Geometry check sheet. Reference: the model listing, model coordinates, mm. A direction names the side the tool comes from. Give positions to 0.01 mm unless a question says otherwise; leave off trailing zeros. Loops run counter-clockwise (first coordinate to the right, second up) from the corner with the lowest first, then second, coordinate; pieces in that order, holes last.
1. Release check for a two-part mould opening along Y. For faces 4 (the cylindrical face through (-43.28, -11.49, 15.55)), 5 (the flat face through (-41, -18, 15)), 6 (the cylindrical face through (-43.306, -11.894, 17.398)), 7 (the flat face through (-42.292, -9, 15)) record: +Y half, -Y half, draft (parallel to the pull), parting line (faces both ways), or undercut.
2. Go/stop test with flat-tipped pins: pin 1 Ø1.2 at (y, z) = (-12, 15) entering from -X; pin 2 Ø3 at (x, y) = (-36.29, -12) entering from -Z; pin 3 Ø1.5 at (y, z) = (-9.5, 14.5) entering from +X; pin 4 Ø1 at (y, z) = (-7.5, 18) entering from -X. Record where each tip stops, or that it passes through.
3. Cross-section at C-C, the plane y = -12. Record the cut outline in (x, z).
4. Cross-section at A-A, the plane z = 18. Record the cut outline in (x, y).
5. Tool access check on faces 1 (the flat face through (-33.292, -12, 12)), 2 (the flat face through (-40.792, -12, 15)), 3 (the flat face through (-42.242, -12, 15)). Record the directions out of +Z, -Z, +X, -X, +Y, -Y that give a thin tool (end or side, any length) a straight path to the whole face; none if there is none.
6. Material ranges on L1, parallel to Y at x = -36.25, z = 11.5; L2, parallel to Z at x = -34, y = -10; L3, parallel to Y at x = -42.95, z = 15, recorded low to high.
7. Cross-section at D-D, the plane z = 15. Record the cut outline in (x, y), plus the area to 3 significant figures.
8. Cross-section at B-B, the plane x = -34.25. Record the cut outline in (y, z), plus the area to 3 significant figures.
from build123d import *

# Parameters (mm, degrees)
SPRING_FRONT_CABLE_CLEVIS_1_SKETCH_W  = 1.5
SPRING_FRONT_CABLE_CLEVIS_1_SKETCH_H  = 12
SPRING_FRONT_CABLE_CLEVIS_1_DEPTH     = 8.1
SPRING_FRONT_CLEVIS_1_LOWER_SKETCH_W  = 7.6
SPRING_FRONT_CLEVIS_1_LOWER_SKETCH_H  = 12
SPRING_FRONT_CLEVIS_1_LOWER_DEPTH     = 1.5
SPRING_FRONT_CLEVIS_1_UPPER_SKETCH_W  = 7.6
SPRING_FRONT_CLEVIS_1_UPPER_SKETCH_H  = 12
SPRING_FRONT_CLEVIS_1_UPPER_DEPTH     = 1.6
FRONT_CLEVIS_SWAGE_HOUSING_1_SKETCH_R = 2.4
FRONT_CLEVIS_SWAGE_HOUSING_1_DEPTH    = 2.1
FRONT_CLEVIS_SWAGE_BORE_1_SKETCH_R    = 0.75
FRONT_CLEVIS_SWAGE_BORE_1_DEPTH       = 2.15
FRONT_CLEVIS_PIN_BORE_1_SKETCH_R      = 1.6
FRONT_CLEVIS_PIN_BORE_1_DEPTH         = 8.3


with BuildPart() as part:
    # Spring Front Cable Clevis 1 sketch → Spring Front Cable Clevis 1 (new body)
    with BuildSketch(Plane.XY.offset(11)):
        with Locations((-41.541651246, -12)):
            Rectangle(SPRING_FRONT_CABLE_CLEVIS_1_SKETCH_W, SPRING_FRONT_CABLE_CLEVIS_1_SKETCH_H)
    extrude(amount=SPRING_FRONT_CABLE_CLEVIS_1_DEPTH)

    # Spring Front Clevis 1 Lower sketch → Spring Front Clevis 1 Lower (add)
    with BuildSketch(Plane.XY.offset(11)):
        with Locations((-37.091651246, -12)):
            Rectangle(SPRING_FRONT_CLEVIS_1_LOWER_SKETCH_W, SPRING_FRONT_CLEVIS_1_LOWER_SKETCH_H)
    extrude(amount=SPRING_FRONT_CLEVIS_1_LOWER_DEPTH)

    # Spring Front Clevis 1 Upper sketch → Spring Front Clevis 1 Upper (add)
    with BuildSketch(Plane.XY.offset(17.5)):
        with Locations((-37.091651246, -12)):
            Rectangle(SPRING_FRONT_CLEVIS_1_UPPER_SKETCH_W, SPRING_FRONT_CLEVIS_1_UPPER_SKETCH_H)
    extrude(amount=SPRING_FRONT_CLEVIS_1_UPPER_DEPTH)

    # Front Clevis Swage Housing 1 sketch → Front Clevis Swage Housing 1 (add)
    with BuildSketch(Plane(origin=(-44.291651246, 0, 0), x_dir=(0, 0, -1), z_dir=(1, 0, 0))):
        with Locations((-15, -12)):
            Circle(FRONT_CLEVIS_SWAGE_HOUSING_1_SKETCH_R)
    extrude(amount=FRONT_CLEVIS_SWAGE_HOUSING_1_DEPTH)

    # Front Clevis Swage Bore 1 sketch → Front Clevis Swage Bore 1 (cut)
    with BuildSketch(Plane(origin=(-44.391651246, 0, 0), x_dir=(0, 0, -1), z_dir=(1, 0, 0))):
        with Locations((-15, -12)):
            Circle(FRONT_CLEVIS_SWAGE_BORE_1_SKETCH_R)
    extrude(amount=FRONT_CLEVIS_SWAGE_BORE_1_DEPTH, mode=Mode.SUBTRACT)

    # Front Clevis Pin Bore 1 sketch → Front Clevis Pin Bore 1 (cut)
    with BuildSketch(Plane.XY.offset(10.9)):
        with Locations((-36.291651246, -12)):
            Circle(FRONT_CLEVIS_PIN_BORE_1_SKETCH_R)
    extrude(amount=FRONT_CLEVIS_PIN_BORE_1_DEPTH, mode=Mode.SUBTRACT)


solid = part.part
Result:
1. face 4: undercut
1. face 5: -Y half
1. face 6: parting line
1. face 7: draft
2. pin 1: stops at x = -42.24
2. pin 2: passes through
2. pin 3: stops at x = -40.79
2. pin 4: stops at x = -42.29
3. outline: (-44.29, 12.6) - (-42.29, 12.6) - (-42.29, 11) - (-37.89, 11) - (-37.89, 12.5) - (-40.79, 12.5) - (-40.79, 17.5) - (-37.89, 17.5) - (-37.89, 19.1) - (-42.29, 19.1) - (-42.29, 17.4) - (-44.29, 17.4) - (-44.29, 15.75) - (-42.24, 15.75) - (-42.24, 14.25) - (-44.29, 14.25) - close; (-34.69, 11) - (-33.29, 11) - (-33.29, 12.5) - (-34.69, 12.5) - close; (-34.69, 17.5) - (-33.29, 17.5) - (-33.29, 19.1) - (-34.69, 19.1) - close
4. outline: (-42.29, -18) - (-33.29, -18) - (-33.29, -6) - (-42.29, -6) - close; hole circle Ø3.2 at (-36.29, -12)
5. face 1: +Z, -Z, +X, +Y, -Y
5. face 2: +X, +Y, -Y
5. face 3: -X
6. L1: y = -18 to -13.6, -10.4 to -6
6. L2: z = 11 to 12.5, 17.5 to 19.1
6. L3: y = -14.4 to -12.75, -11.25 to -9.6
7. outline: (-44.29, -14.4) - (-42.29, -14.4) - (-42.29, -18) - (-40.79, -18) - (-40.79, -6) - (-42.29, -6) - (-42.29, -9.6) - (-44.29, -9.6) - (-44.29, -11.25) - (-42.24, -11.25) - (-42.24, -12.75) - (-44.29, -12.75) - close
7. area: 24.5 mm2
8. outline: (-18, 11) - (-6, 11) - (-6, 12.5) - (-18, 12.5) - close; (-18, 17.5) - (-6, 17.5) - (-6, 19.1) - (-18, 19.1) - close
8. area: 37.2 mm2
